Check sheet for the modelled part. Datum: model origin and axes. Units: mm. A direction names the side the tool comes from. Round coordinates to 2 decimals unless told otherwise and drop trailing zeros. Write each loop counter-clockwise with the first axis right and the second up, starting at its lowest first coordinate (ties: lowest second). Pieces come first, ordered by that corner, then holes. Notation, with made-up numbers: (39, -23.75) -> (60, -23.75) arc R28 cw to (60, 12.25) -> close; hole circle Ø9 at (60, 75.25). An arc over 180 degrees is marked (long way). One line per item, written item: value.
from build123d import *

# Parameters (mm, degrees)
SKETCH1_R           = 17
SKETCH1_R_2         = 12.5
BOSS_EXTRUDE1_DEPTH = 29
SKETCH2_W           = 8
SKETCH2_H           = 5
CUT_EXTRUDE2_DEPTH  = 28
FILLET3_R           = 4
FILLET4_R           = 4
SKETCH3_R           = 1.5
CUT_EXTRUDE4_DEPTH  = 47.411205606


with BuildPart() as part:
    # Sketch1 → Boss-Extrude1 (new body)
    with BuildSketch(Plane.XY):
        with Locations(Location((0, 0, 0), (0, 0, 180))):
            Circle(SKETCH1_R)
        with Locations(Location((0, 0, 0), (0, 0, 180))):
            Circle(SKETCH1_R_2, mode=Mode.SUBTRACT)
    extrude(amount=BOSS_EXTRUDE1_DEPTH)

    # Sketch2 → Cut-Extrude2 (cut)
    with BuildSketch(Plane.XY.offset(29)):
        with Locations((0, 12.5)):
            Rectangle(SKETCH2_W, SKETCH2_H)
    extrude(amount=-CUT_EXTRUDE2_DEPTH, mode=Mode.SUBTRACT)

    # Fillet3
    fillet3_edges = [part.edges().sort_by_distance(p)[0] for p in [
        (-4, 13.421359641, 1),
    ]]
    fillet(fillet3_edges, radius=FILLET3_R)

    # Fillet4
    fillet4_edges = [part.edges().sort_by_distance(p)[0] for p in [
        (4, 13.421359641, 1),
    ]]
    fillet(fillet4_edges, radius=FILLET4_R - 0.0001)  # a hair under: the kernel refuses the full size

    # Sketch3 → Cut-Extrude4 (cut, through all)
    with BuildSketch(Plane(origin=(0, 15, 0), x_dir=(-1, 0, 0), z_dir=(0, -1, 0))):
        with Locations(Location((0, -9, 0), (0, 0, 90))):
            Circle(SKETCH3_R)
    extrude(amount=-CUT_EXTRUDE4_DEPTH, mode=Mode.SUBTRACT)


solid = part.part
Item 1: Sectioned sample at C-C on z = 24. Enter the section's corners in (x, y), and give its area (3 significant figures).
Answer:
outline: circle Ø34 at (0, 0); hole (-4, 11.84) arc R12.5 ccw (long way) to (4, 11.84) -> (4, 15) -> (-4, 15) -> close
area: 395 mm^2
Item 2: Mould release check, pull along Y, two halves, no side actions. Record for faces 4 (the cylindrical face through (2.213, -16.855, 14.297)), 5 (the flat face through (8, -10, 29)), 6 (the flat face through (4, 13, 17)): pulls with the +Y half, pulls with the -Y half, needs draft (parallel to the pull), parting line crosses it, or undercut.
Answer:
face 4: parting line crosses it
face 5: needs draft
face 6: undercut
Item 3: Thickness scan on line 1 (Y direction, x = 0, z = 18); line 2 (X direction, y = 9, z = 19.5); line 3 (X direction, y = -8.5, z = 2.5). Record the ranges inside material, lowest first.
Answer:
line 1: y = -17 to -12.5, 15 to 17
line 2: x = -14.42 to -8.67, 8.67 to 14.42
line 3: x = -14.72 to -9.17, 9.17 to 14.72
Item 4: Sectioned sample at D-D on x = -1. Enter the section's corners in (y, z).
Answer:
outline: (-16.97, 0) -> (-12.46, 0) -> (-12.46, 29) -> (-16.97, 29) -> close; (12.46, 0) -> (16.97, 0) -> (16.97, 7.88) -> (15, 7.88) -> (15, 1.13) -> (12.46, 1.13) -> close; (15, 10.12) -> (16.97, 10.12) -> (16.97, 29) -> (15, 29) -> close
Item 5: Sectioned sample at B-B on x = 7.5. Enter the section's corners in (y, z), and give its area (3 significant figures).
Answer:
outline: (-15.26, 0) -> (-10, 0) -> (-10, 29) -> (-15.26, 29) -> close; (10, 0) -> (15.26, 0) -> (15.26, 29) -> (10, 29) -> close
area: 305 mm^2
Item 6: Depth check by flat-ended pin: P1, Ø8, axis at y = -10.5, z = 5.5, coming from the +X side; P2, Ø2.5, axis at x = 0, z = 9, coming from the +Y side; P3, Ø3, axis at x = 12.5, z = 12, coming from the +Y side. Enter the tip coordinate at first touch or a pass-through.
Answer:
P1: stops at x = 15.71
P2: stops at y = -12.44
P3: stops at y = 12.96
Item 7: Sectioned sample at A-A on y = 0. Enter the section's corners in (x, z), and give its area (3 significant figures).
Answer:
outline: (-17, 0) -> (-12.5, 0) -> (-12.5, 29) -> (-17, 29) -> close; (12.5, 0) -> (17, 0) -> (17, 29) -> (12.5, 29) -> close
area: 261 mm^2
Item 8: Tool access check on faces 1 (the cylindrical face through (0.07, 15.99, 10.5)), 2 (the flat face through (-4, 13, 17)), 3 (the cylindrical face through (1.627, -12.394, 14.297)). Record the directions out of +Z, -Z, +X, -X, +Y, -Y that give a thin tool (end or side, any length) a straight path to the whole face; none if there is none.
Answer:
face 1: +Y
face 2: +Z
face 3: +Z, -Z
